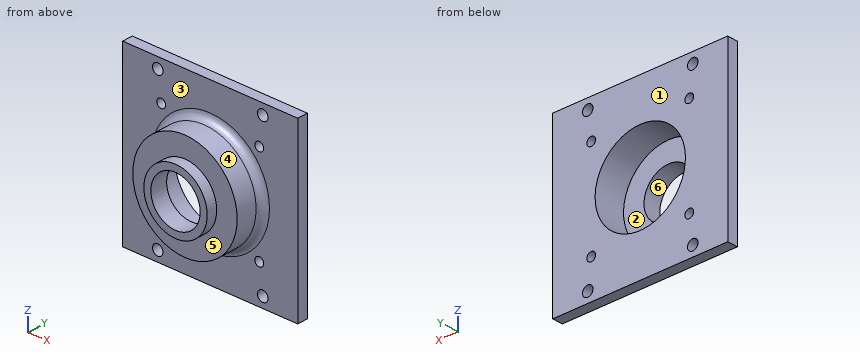
from build123d import *

# Parameters (mm, degrees)
BOSS_EXTRUDE1_START = -3
SKETCH3_W           = 50
SKETCH3_H           = 50
SKETCH3_R           = 14.9
BOSS_EXTRUDE1_DEPTH = 3
SKETCH4_R           = 1.25
SKETCH4_R_2         = 1.5
CUT_EXTRUDE1_DEPTH  = 39.026306684
FILLET1_R           = 2


with BuildPart() as part:
    # Sketch2 → Revolve-Thin1 (revolve)
    with BuildSketch(Plane.XY, mode=Mode.PRIVATE) as revolve_thin1_sk:
        Polygon((7.05, 0), (7.05, 5), (12.9, 5), (12.9, 14), (14.9, 14), (14.9, 3), (9.05, 3), (9.05, 0), align=None)
    revolve(revolve_thin1_sk.sketch.rotate(Axis((0, 56.528570812, 0), (0, -1, 0)), 90), axis=Axis((0, 56.528570812, 0), (0, -1, 0)))

    # Sketch3 → Boss-Extrude1 (add)
    with BuildSketch(Plane(origin=(0, 14, 0), x_dir=(1, 0, 0), z_dir=(0, 1, 0)).offset(BOSS_EXTRUDE1_START)):
        Rectangle(SKETCH3_W, SKETCH3_H)
        with Locations(Location((0, 0, 0), (0, 0, 270))):
            Circle(SKETCH3_R, mode=Mode.SUBTRACT)
    extrude(amount=BOSS_EXTRUDE1_DEPTH)

    # Sketch4 → Cut-Extrude1 (cut, through all)
    with BuildSketch(Plane(origin=(0, 14, 0), x_dir=(1, 0, 0), z_dir=(0, 1, 0))):
        with Locations(Location((14, 14, 0), (0, 0, 270))):
            Circle(SKETCH4_R)
        with Locations(Location((-14, 14, 0), (0, 0, 270))):
            Circle(SKETCH4_R)
        with Locations(Location((-14, -14, 0), (0, 0, 270))):
            Circle(SKETCH4_R)
        with Locations(Location((14, -14, 0), (0, 0, 270))):
            Circle(SKETCH4_R)
        with Locations(Location((-15, 22, 0), (0, 0, 270))):
            Circle(SKETCH4_R_2)
        with Locations(Location((15, 22, 0), (0, 0, 270))):
            Circle(SKETCH4_R_2)
        with Locations(Location((15, -22, 0), (0, 0, 270))):
            Circle(SKETCH4_R_2)
        with Locations(Location((-15, -22, 0), (0, 0, 270))):
            Circle(SKETCH4_R_2)
    extrude(amount=-CUT_EXTRUDE1_DEPTH, mode=Mode.SUBTRACT)

    # Fillet1
    fillet1_edges = [part.edges().sort_by_distance(p)[0] for p in [
        (0, 11, -14.9),
    ]]
    fillet(fillet1_edges, radius=FILLET1_R)


solid = part.part
Work out the finished part from the listing and answer in its coordinate system (mm). Face numbers are marked on the shaded views. A direction names the side the tool comes from. Coordinates: 2 decimals unless noted, no trailing zeros. Loops run counter-clockwise (first coordinate to the right, second up) from the corner with the lowest first, then second, coordinate; pieces in that order, holes last. Notation, with made-up numbers: (68.25, 52.5) -> (119.25, 52.5) arc R12 ccw to (119.25, 56.5) -> close; hole circle Ø10 at (-11.5, -19.5). An arc over 180 degrees is marked (long way). Answer as CSV lines item,"result".
1) The part is cut by section D-D (x = 21). Give the vertices of the cut face in (y, z).
A:
outline,"(11, -25) -> (14, -25) -> (14, 25) -> (11, 25) -> close"
2) For the marked faces 1, 2 and 3, determine the directions among +Z, -Z, +X, -X, +Y, -Y from which every point of the face is accessible in a straight line to the end or side of a thin tool.
A:
face 1,"+Z, -Z, +X, -X, +Y"
face 2,"+Y"
face 3,"-Y"
3) Flat-ended cylindrical pins translate along their axes: pin 1 (8 mm diameter, centred on y = 2.5, z = 17.5, fed in from +X); pin 2 (2 mm diameter, centred on x = 4.5, y = 9, fed in from -Z); pin 3 (1 mm diameter, centred on y = 4, z = 4, fed in from +X). Find the tip coordinate at first contact, or state that the pin passes through.
A:
pin 1,"stops at x = 6.24"
pin 2,"stops at z = -14.56"
pin 3,"stops at x = 14.48"
4) For a pull along Z with two mould halves and no side action, classify the marked faces 4, 5 and 6 as released by +Z, released by -Z, zero draft, split by the parting line, or undercut.
A:
face 4,"split by the parting line"
face 5,"zero draft"
face 6,"undercut"
5) Straight lines are drawn through the part: probe 1 along X at (y, z) = (12.4, -22); probe 2 along X at (y, z) = (12, -14); probe 3 along Z at (x, y) = (14.5, 13.25). For each, find the intervals that lie inside material, in ascending order.
A:
probe 1,"x = -25 to -16.5, -13.5 to 13.5, 16.5 to 25"
probe 2,"x = -25 to -15.25, -12.75 to 12.75, 15.25 to 25"
probe 3,"z = -25 to -23.41, -20.59 to -15.15, -12.85 to 12.85, 15.15 to 20.59, 23.41 to 25"
6) The part is cut by section A-A (x = 0). Give the vertices of the cut face in (y, z).
A:
outline,"(0, -9.05) -> (3, -9.05) -> (3, -14.9) -> (9, -14.9) arc R2 cw to (11, -16.9) -> (11, -25) -> (14, -25) -> (14, -12.9) -> (5, -12.9) -> (5, -7.05) -> (0, -7.05) -> close; (0, 7.05) -> (5, 7.05) -> (5, 12.9) -> (14, 12.9) -> (14, 25) -> (11, 25) -> (11, 16.9) arc R2 cw to (9, 14.9) -> (3, 14.9) -> (3, 9.05) -> (0, 9.05) -> close"
7) The part is cut by section C-C (y = 5.75). Give the vertices of the cut face in (x, z).
A:
outline,"circle Ø29.8 at (0, 0); hole circle Ø25.8 at (0, 0)"
8) The part is cut by section B-B (z = -22). Give the vertices of the cut face in (x, y), and give its area (3 significant figures).
A:
outline,"(-25, 11) -> (-16.5, 11) -> (-16.5, 14) -> (-25, 14) -> close; (-13.5, 11) -> (13.5, 11) -> (13.5, 14) -> (-13.5, 14) -> close; (16.5, 11) -> (25, 11) -> (25, 14) -> (16.5, 14) -> close"
area,"132 mm²"
